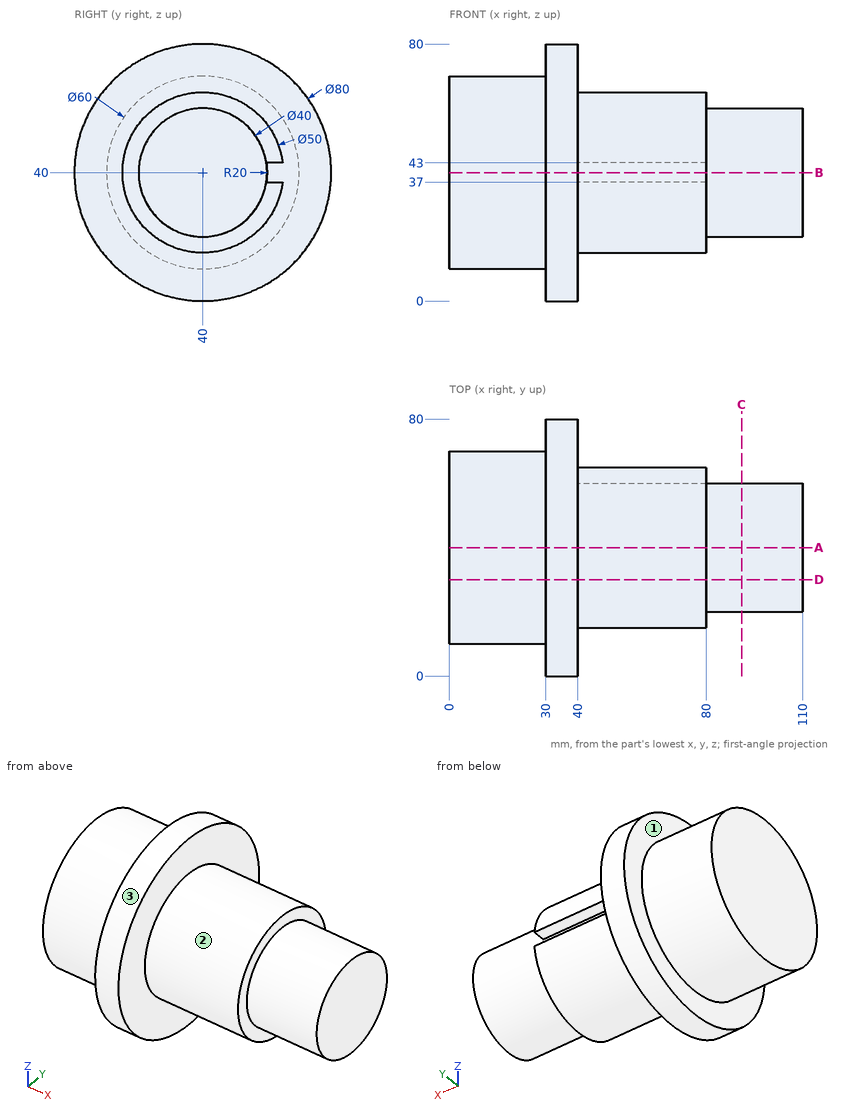
Answer from the drawing. Dimensions are ordinates in mm from the lowest x, y and z of the part. A direction names the side the tool comes from. Round coordinates to 2 decimals unless told otherwise and drop trailing zeros. Loops run counter-clockwise (first coordinate to the right, second up) from the corner with the lowest first, then second, coordinate; pieces in that order, holes last.
1) A cutting plane is placed at D-D on y = 30. Determine the outline of the cut face in (x, z).
Outcome:
outline: (0, 11.72) - (30, 11.72) - (30, 1.27) - (40, 1.27) - (40, 17.09) - (80, 17.09) - (80, 22.68) - (110, 22.68) - (110, 57.32) - (80, 57.32) - (80, 62.91) - (40, 62.91) - (40, 78.73) - (30, 78.73) - (30, 68.28) - (0, 68.28) - close
2) A cutting plane is placed at B-B on z = 40. Determine the outline of the cut face in (x, y).
Outcome:
outline: (0, 10) - (30, 10) - (30, 0) - (40, 0) - (40, 15) - (80, 15) - (80, 20) - (110, 20) - (110, 60) - (40, 60) - (40, 80) - (30, 80) - (30, 70) - (0, 70) - close
3) Consider line 1 (X direction, y = 56.5, z = 57.5); line 2 (X direction, y = 27.5, z = 71.5); line 3 (Z direction, x = 64.5, y = 59.5). Determine where each line is inside the solid, lowest interval first.
Outcome:
line 1: x = 0 to 80
line 2: x = 30 to 40
line 3: z = 24.36 to 55.64
4) A cutting plane is placed at C-C on x = 91. Determine the outline of the cut face in (y, z), plus the area to 3 significant figures.
Outcome:
outline: circle Ø40 at (40, 40)
area: 1,260 mm2
5) Given P1, Ø6, axis at x = 43.5, y = 49.5, coming from the +Z side; P2, Ø4, axis at y = 40.5, z = 11.5, coming from the -X side; P3, Ø3, axis at x = 11.5, z = 26.5, coming from the +Y side; P4, Ø1.5, axis at x = 26.5, y = 30.5, coming from the +Z side, each flat-ended and moving along its own axis, determine where each tip first touches the part or whether it passes through.
Outcome:
P1: stops at z = 64.14
P2: stops at x = 0
P3: stops at y = 67.5
P4: stops at z = 68.7
6) A cutting plane is placed at A-A on y = 40. Determine the outline of the cut face in (x, z).
Outcome:
outline: (0, 10) - (30, 10) - (30, 0) - (40, 0) - (40, 15) - (80, 15) - (80, 20) - (110, 20) - (110, 60) - (80, 60) - (80, 65) - (40, 65) - (40, 80) - (30, 80) - (30, 70) - (0, 70) - close
7) For the marked faces 1, 2 and 3, determine the directions among +Z, -Z, +X, -X, +Y, -Y from which every point of the face is accessible in a straight line to the end or side of a thin tool.
Outcome:
face 1: -X
face 2: +X
face 3: +X, -X
